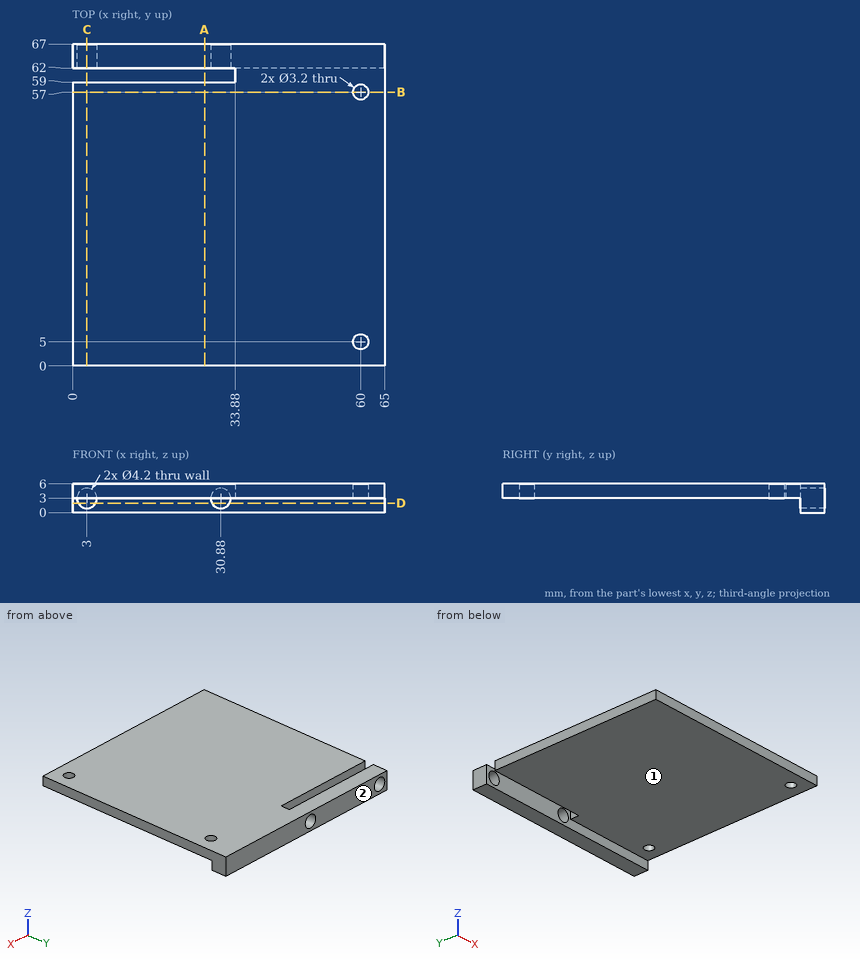
Source: three-view drawing plus pictorial views. Frame: mm from the lowest corner of the part. A direction names the side the tool comes from. Give positions to 0.01 mm unless a question says otherwise; leave off trailing zeros. Write each loop counter-clockwise with the first axis right and the second up, starting at its lowest first coordinate (ties: lowest second). Pieces come first, ordered by that corner, then holes.
(1) Ray query, line 1 (X direction, y = 64, z = 3); line 2 (Z direction, x = 3, y = 64.2); line 3 (X direction, y = 5, z = 3.85). Return the intervals inside material, ascending.
(2) Cut plane D-D, the plane z = 2. Return loops of the section in (x, y).
(3) Cut plane B-B, the plane y = 57. Return loops of the section in (x, z).
(4) Cut plane A-A, the plane x = 27.5. Return loops of the section in (y, z), then the cut area to 3 significant figures.
(5) First-contact query: P1, Ø1.5, axis at y = 61, z = 5, coming from the -X side; P2, Ø1.5, axis at x = 8.5, z = 3.5, coming from the -Y side; P3, Ø1.8, axis at x = 43.5, z = 2, coming from the -Y side; P4, Ø3.5, axis at x = 60, y = 57, coming from the -Z side. Flat tips, straight axial feed; report the tip coordinate or a pass-through.
(6) Access query for the marked faces 1 and 2. Directions: +Z, -Z, +X, -X, +Y, -Y. A direction counts if a zero-diameter tool reaches every point of the face in a straight line with its end or side. Return the directions, or none.
(7) Cut plane C-C, the plane x = 3. Return loops of the section in (y, z), then the cut area to 3 significant figures.
Values follow:
1. line 1: x = 0 to 0.9, 5.1 to 28.78, 32.98 to 65
1. line 2: z = 0 to 0.9, 5.1 to 6
1. line 3: x = 0 to 58.4, 61.6 to 65
2. outline: (0, 62) - (1.15, 62) - (1.15, 67) - (0, 67) - close; (4.85, 62) - (29.03, 62) - (29.03, 67) - (4.85, 67) - close; (32.73, 62) - (65, 62) - (65, 67) - (32.73, 67) - close
3. outline: (0, 3) - (58.4, 3) - (58.4, 6) - (0, 6) - close; (61.6, 3) - (65, 3) - (65, 6) - (61.6, 6) - close
4. outline: (0, 3) - (59, 3) - (59, 6) - (0, 6) - close; (62, 0) - (67, 0) - (67, 6) - (62, 6) - close
4. area: 207 mm2
5. P1: stops at x = 33.88
5. P2: stops at y = 0
5. P3: stops at y = 62
5. P4: stops at z = 3
6. face 1: -Z, +X, -X, -Y
6. face 2: +Z, -Z, +X, -X, +Y
7. outline: (0, 3) - (59, 3) - (59, 6) - (0, 6) - close; (62, 0) - (67, 0) - (67, 0.9) - (62, 0.9) - close; (62, 5.1) - (67, 5.1) - (67, 6) - (62, 6) - close
7. area: 186 mm2
